Autodesk Inventor part; units mm, degrees
ref_plane "YZ Plane" through (0, 0, 0) normal (1, 0, 0) x (0, 1, 0)
ref_plane "XZ Plane" through (0, 0, 0) normal (0, 1, 0) x (-1, 0, 0)
ref_plane "XY Plane" through (0, 0, 0) normal (0, 0, 1) x (1, 0, 0)
sketch "Sketch1" plane through (0, 0, 0) normal (0, 0, 1) x (1, 0, 0)
  line L0 (-20, 20) -> (20, 20)
  line L1 (20, 20) -> (20, -20)
  line L2 (20, -20) -> (-20, -20)
  line L3 (-20, -20) -> (-20, 20)
  point P0 (0, 0)
  point P1 (-20, 0)
  point P2 (0, 20)
  dimension "d0" = 40
  dimension "d1" = 40
extrude "Extrusion1" add sketch "Sketch1" along normal blind 20
sketch "Sketch2" plane through (-20, -20, 0) normal (0, -1, 0) x (1, 0, 0)
  line L0 (0, 0) -> (40, 0)
  line L1 (0, 0) -> (0, 20)
  line L2 (40, 0) -> (0, 0)
  line L3 (0, 0) -> (0, 3)
  line L4 (0, 3) -> (40, 3)
  line L5 (40, 3) -> (40, 0)
  line L6 (40, 0) -> (0, 0)
  line L7 (32, 0) -> (32, 3)
  line L8 (32, 3) -> (33.7321, 0)
  line L9 (32, 3) -> (30.2679, 0)
  point P0 (20, 0)
  point P1 (40, 1.5)
  dimension "d4" = 3
  dimension "d5" = 8
  dimension "d6" = 30
  dimension "d7" = 30
extrude "Extrusion2" cut sketch "Sketch2" against normal through all contours L9 L7 L0 | L7 L8 L0
pattern_linear "Rectangular Pattern1" count 4 spacing 8 along (-1, 0, 0) of "Extrusion2"
ref_plane "Work Plane1" through (-20, 0, 20) normal (0, -1, 0) x (1, 0, 0)
ref_plane "Work Plane2" through (0, -20, 0) normal (1, 0, 0) x (0, 0, -1)
pattern_circular "Circular Pattern1" count 2 over 90 about axis through (0, 0, 20) along (0, 0, 1) of "Extrusion2", "Rectangular Pattern1"
chamfer "Chamfer1" distance 3 angle 30 5 edges at (16.866, 20, 0) (8, 20, 0) (0, 20, 0) (-8, 20, 0) (-16.866, 20, 0) measured on face at (-1.3333, 20, 14.3333)
chamfer "Chamfer2" distance 3 angle 30 5 edges at (-20, 16.0003, 0) (-20, 8, 0) (-20, 0, 0) (-20, -8, 0) (-20, -16.866, 0) measured on face at (-20, -1.3333, 14.3333)
chamfer "Chamfer3" distance 3 angle 30 5 edges at (-16.0003, -20, 0) (-8, -20, 0) (0, -20, 0) (8, -20, 0) (16.866, -20, 0) measured on face at (1.3333, -20, 14.3333)
chamfer "Chamfer4" distance 3 angle 30 5 edges at (20, -16.0003, 0) (20, -8, 0) (20, 8, 0) (20, 0, 0) (20, 16.0003, 0) measured on face at (20, 1.3333, 14.3333)
properties part number "LI0013-FOOT"
Can you work these out from the model? Positions are in its coordinate system, mm. A direction names the side the tool comes from. Coordinates: 2 decimals unless noted, no trailing zeros. Write each loop counter-clockwise with the first axis right and the second up, starting at its lowest first coordinate (ties: lowest second). Pieces come first, ordered by that corner, then holes. Notation, with made-up numbers: (2.25, 68.25) - (9.25, 68.25) arc R26 ccw to (9.25, 105.25) - close; hole circle Ø4 at (-7, 84.25). An arc over 180 degrees is marked (long way). Return JSON: item names as keys, results as strings.
Q1. If we section it at B-B (x = -0.5): Please give me the cut outline in (y, z).
Computed values:
{"outline": "(-20, 3) - (-18.27, 0) - (-13.73, 0) - (-12, 3) - (-10.27, 0) - (-5.73, 0) - (-4, 3) - (-2.27, 0) - (2.27, 0) - (4, 3) - (5.73, 0) - (10.27, 0) - (12, 3) - (13.73, 0) - (18.27, 0) - (20, 3) - (20, 20) - (-20, 20) - close"}
Q2. Please list where these lines run through material, in increasing order: L1, parallel to X at y = -2, z = 1.75; L2, parallel to Y at x = 3.5, z = 2.5; L3, parallel to Y at x = -16, z = 1.5. Write a range as from..to.
Computed values:
{"L1": "x = -19.28..-12.72, -11.28..-4.72, -3.28..3.28, 4.72..11.28, 12.72..19.28", "L2": "y = -19.71..-12.29, -11.71..-4.29, -3.71..3.71, 4.29..11.71, 12.29..19.71", "L3": "y = -19.13..-12.87, -11.13..-4.87, -3.13..3.13, 4.87..11.13, 12.87..19.13"}
Q3. Thinking about a two-plate mould opening in Y: for faces 1 (the flat face through (-7.944, 3.146, 1.521)), 2 (the flat face through (-19.122, 16.056, 1.479)), 3 (the flat face through (0, -20, 11)), which applies, +Y half, -Y half, draft (parallel to the pull), parting line (faces both ways), or undercut?
Computed values:
{"face 1": "undercut", "face 2": "draft", "face 3": "-Y half"}
Q4. On a 3-axis mill with a long thin cutter (end or side, diameter ignored), from which of +Z, -Z, +X, -X, +Y, -Y can I reach the whole of each face in a straight line? I mean faces 4 (the flat face through (12.854, 7.944, 1.521)), 5 (the flat face through (19.122, -8.056, 1.479)), 6 (the flat face through (8.056, -12.854, 1.521)). Say none if no direction works.
Computed values:
{"face 4": "-Z, +Y, -Y", "face 5": "-Z, +X, +Y, -Y", "face 6": "-Z, +X, -X"}
Q5. If we section it at A-A (y = -13): Please give me the cut outline in (x, z), then the cut area to 3 significant figures.
Computed values:
{"outline": "(-20, 3) - (-19, 1.27) - (-13, 1.27) - (-12, 3) - (-11, 1.27) - (-5, 1.27) - (-4, 3) - (-3, 1.27) - (3, 1.27) - (4, 3) - (5, 1.27) - (11, 1.27) - (12, 3) - (13, 1.27) - (19, 1.27) - (20, 3) - (20, 20) - (-20, 20) - close", "area": "741 mm2"}
